For this review, take the finished solid that the model builds, in its own axes (mm). Face numbers are marked on the shaded views. A direction names the side the tool comes from. Round coordinates to 2 decimals unless told otherwise and drop trailing zeros. Write each loop counter-clockwise with the first axis right and the second up, starting at its lowest first coordinate (ties: lowest second). Pieces come first, ordered by that corner, then holes. Notation, with made-up numbers: M 86.5,9 L 142.5,9 A15 cw 142.5,26 Z; hole C 88.25,71 d11. An arc over 180 degrees is marked long. Answer in a Markdown table with one row per item.
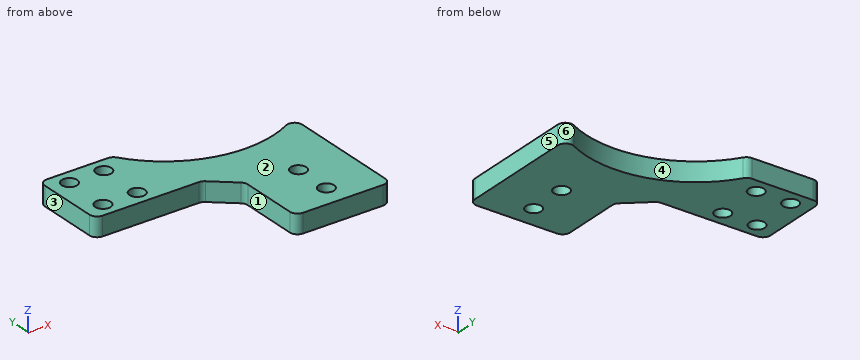
```python
from build123d import *

# Parameters (mm, degrees)
EXTRUDE_1_DEPTH          = 2.5
FILLET_1_R               = 2
FILLET_2_R               = 2
SKETCH_2_R               = 2.025
CUT_EXTRUDE_1_DEPTH      = 6
SKETCH_3_W               = 25
SKETCH_3_H               = 6
CUT_EXTRUDE_2_DEPTH      = 6
FILLET_3_R               = 2
SKETCH_4_R               = 2.025
CUT_EXTRUDE_3_DEPTH      = 1
CUT_EXTRUDE_3_DEPTH_BACK = 6
SKETCH_5_R               = 2.025
CUT_EXTRUDE_4_DEPTH      = 1
CUT_EXTRUDE_4_DEPTH_BACK = 6


with BuildPart() as part:
    # 草图1 → 凸台-拉伸1 (new body, symmetric)
    with BuildSketch(Plane.XY):
        with BuildLine():
            Line((0, 0), (0, -24))
            Line((0, -24), (25, -24))
            Line((25, -24), (25, 17.256579859))
            ThreePointArc((25, 17.256579859), (2.677238779, 12.836790892), (-15.885361498, 26))
            Line((-15.885361498, 26), (-35, 26))
            Line((-35, 26), (-35, 6))
            Line((-35, 6), (-7, 6))
            Line((-7, 6), (0, 0))
        make_face()
    extrude(amount=EXTRUDE_1_DEPTH, both=True)

    # 圆角1
    fillet_1_edges = [part.edges().sort_by_distance(p)[0] for p in [
        (-7, 6, 0),
        (-35, 6, 0),
        (-35, 26, 0),
        (25, -24, 0),
        (0, -24, 0),
        (0, 0, 0),
    ]]
    fillet(fillet_1_edges, radius=FILLET_1_R)

    # 圆角2
    fillet_2_edges = [part.edges().sort_by_distance(p)[0] for p in [
        (-15.885361498, 26, 0),
        (25, 17.256579859, 0),
    ]]
    fillet(fillet_2_edges, radius=FILLET_2_R)

    # 草图2 → 切除-拉伸1 (cut, through all)
    with BuildSketch(Plane.XY.offset(2.5)):
        with Locations((12.5, -2)):
            Circle(SKETCH_2_R)
        with Locations((12.5, -12)):
            Circle(SKETCH_2_R)
    extrude(amount=-CUT_EXTRUDE_1_DEPTH, mode=Mode.SUBTRACT)

    # 草图3 → 切除-拉伸2 (cut, through all)
    with BuildSketch(Plane.XY.offset(2.5)):
        with Locations((12.5, -21)):
            Rectangle(SKETCH_3_W, SKETCH_3_H)
    extrude(amount=-CUT_EXTRUDE_2_DEPTH, mode=Mode.SUBTRACT)

    # 圆角3
    fillet_3_edges = [part.edges().sort_by_distance(p)[0] for p in [
        (0, -18, 0),
        (25, -18, 0),
    ]]
    fillet(fillet_3_edges, radius=FILLET_3_R)

    # 草图4 → 切除-拉伸3 (cut, two sides)
    with BuildSketch(Plane.XY.offset(2.5)) as cut_extrude_3_sk:
        with Locations((-30, 22)):
            Circle(SKETCH_4_R)
        with Locations((-30, 10)):
            Circle(SKETCH_4_R)
    extrude(amount=CUT_EXTRUDE_3_DEPTH, mode=Mode.SUBTRACT)
    extrude(cut_extrude_3_sk.sketch, amount=-CUT_EXTRUDE_3_DEPTH_BACK, mode=Mode.SUBTRACT)

    # 草图5 → 切除-拉伸4 (cut, two sides)
    with BuildSketch(Plane.XY.offset(2.5)) as cut_extrude_4_sk:
        with Locations((-21, 10)):
            Circle(SKETCH_5_R)
        with Locations((-21, 22)):
            Circle(SKETCH_5_R)
    extrude(amount=CUT_EXTRUDE_4_DEPTH, mode=Mode.SUBTRACT)
    extrude(cut_extrude_4_sk.sketch, amount=-CUT_EXTRUDE_4_DEPTH_BACK, mode=Mode.SUBTRACT)


solid = part.part
```
Q1. Machinability: for the marked faces 1 and 2, which of the approach directions +Z, -Z, +X, -X, +Y, -Y give a long, thin tool a straight path to every point of the face, cutting with its end or side? Answer none if there is none.
Found:
| item | result |
|---|---|
| face 1 | +Z, -Z, -X, -Y |
| face 2 | +Z, +X, -X, +Y, -Y |
Q2. Mouldability with a two-part tool opening along X and no side actions: class the marked faces 3, 4, 5 and 6 as +X half, -X half, draft (parallel to the pull), parting line (faces both ways), or undercut.
Found:
| item | result |
|---|---|
| face 3 | -X half |
| face 4 | undercut |
| face 5 | +X half |
| face 6 | undercut |
Q3. Insertion check: P1, Ø2.5, axis at x = -23.5, z = -1, coming from the -Y side; P2, Ø2.5, axis at y = -7.5, z = 0, coming from the -X side. Each pin has a flat end and moves straight along its axis. Give the tip position at first contact, or say it passes through.
Found:
| item | result |
|---|---|
| P1 | y = 6 |
| P2 | x = 0 |
Q4. Take a section at D-D (x = 12.5). State the section outline as (y, z) points (3 decimals), then the cut area to 3 significant figures.
Found:
| item | result |
|---|---|
| outline | M -18,-2.5 L -14.025,-2.5 L -14.025,2.5 L -18,2.5 Z; M -9.975,-2.5 L -4.025,-2.5 L -4.025,2.5 L -9.975,2.5 Z; M 0.025,-2.5 L 12.452,-2.5 L 12.452,2.5 L 0.025,2.5 Z |
| area | 112 mm² |
Q5. For probe 1 along Y at (x, z) = (-21, -0.85) (3 decimals); probe 2 along Y at (x, z) = (12.5, -0.75) (3 decimals); probe 3 along X at (y, z) = (-8.5, 1.4), list the stretches that pass through material, from the lowest coordinate up.
Found:
| item | result |
|---|---|
| probe 1 | 6 to 7.975, 12.025 to 19.975, 24.025 to 26 |
| probe 2 | -18 to -14.025, -9.975 to -4.025, 0.025 to 12.452 |
| probe 3 | 0 to 25 |
Q6. Take a section at A-A (y = -2). State the section outline as (x, z) points (3 decimals), then the cut area to 3 significant figures.
Found:
| item | result |
|---|---|
| outline | M 0,-2.5 L 10.475,-2.5 L 10.475,2.5 L 0,2.5 Z; M 14.525,-2.5 L 25,-2.5 L 25,2.5 L 14.525,2.5 Z |
| area | 105 mm² |
Q7. Take a section at C-C (z = 0.6). State the section outline as (x, y) points (3 decimals).
Found:
| item | result |
|---|---|
| outline | M -35,8 A2 ccw -33,6 L -7.74,6 A2 cw -6.438,5.519 L -0.698,0.599 A2 cw 0,-0.92 L 0,-16 A2 ccw 2,-18 L 23,-18 A2 ccw 25,-16 L 25,13.721 A2 ccw 22.071,15.492 A28.8 cw -15.316,25.104 A2 ccw -16.983,26 L -33,26 A2 ccw -35,24 Z; hole C -30,10 d4.05; hole C -30,22 d4.05; hole C -21,10 d4.05; hole C -21,22 d4.05; hole C 12.5,-12 d4.05; hole C 12.5,-2 d4.05 |
Q8. Take a section at B-B (y = 10). State the section outline as (x, z) points (3 decimals).
Found:
| item | result |
|---|---|
| outline | M -35,-2.5 L -32.025,-2.5 L -32.025,2.5 L -35,2.5 Z; M -27.975,-2.5 L -23.025,-2.5 L -23.025,2.5 L -27.975,2.5 Z; M -18.975,-2.5 L 25,-2.5 L 25,2.5 L -18.975,2.5 Z |
